Source: CAD feature listing. Evaluate the final solid. Frame: model axes, mm. A direction names the side the tool comes from. Round coordinates to 2 decimals unless told otherwise and drop trailing zeros. Loops run counter-clockwise (first coordinate to the right, second up) from the corner with the lowest first, then second, coordinate; pieces in that order, holes last. Notation, with made-up numbers: M -23.5,16.5 L -8.5,16.5 A27 ccw -8.5,55.5 Z; hole C 62.25,-11.75 d7. An arc over 180 degrees is marked long. One line per item, written item: value.
from build123d import *

# Parameters (mm, degrees)
ESBO_O1_W             = 8
ESBO_O1_H             = 8
CORTE_EXTRUS_O1_DEPTH = 46


with BuildPart() as part:
    # Sketch1 → Revolve1 (revolve)
    with BuildSketch(Plane.XY):
        with BuildLine():
            Line((0, -20), (0, -122))
            ThreePointArc((0, -122), (0.146446609, -122.353553391), (0.5, -122.5))
            Line((0.5, -122.5), (9.616336506, -122.5))
            ThreePointArc((9.616336506, -122.5), (9.920717221, -122.39667667), (10.099299419, -122.129409523))
            Line((10.099299419, -122.129409523), (12.679491924, -112.5))
            Line((12.679491924, -112.5), (22.320508076, -112.5))
            Line((22.320508076, -112.5), (24.900700581, -122.129409523))
            ThreePointArc((24.900700581, -122.129409523), (25.079282779, -122.39667667), (25.383663494, -122.5))
            Line((25.383663494, -122.5), (34.5, -122.5))
            ThreePointArc((34.5, -122.5), (34.853553391, -122.353553391), (35, -122))
            Line((35, -122), (35, -50))
            Line((35, -50), (44.5, -50))
            ThreePointArc((44.5, -50), (44.853553391, -49.853553391), (45, -49.5))
            Line((45, -49.5), (45, -10))
            Line((45, -10), (2.5, -10))
            Line((2.5, -10), (0, -20))
        make_face()
    revolve(axis=Axis((0, 0, 0), (1, 0, 0)))

    # Esboço1 → Corte-extrusão1 (cut, through all)
    with BuildSketch(Plane.ZY):
        with Locations((0, -10)):
            Rectangle(ESBO_O1_W, ESBO_O1_H)
    extrude(amount=-CORTE_EXTRUS_O1_DEPTH, mode=Mode.SUBTRACT)


solid = part.part
1. Reachability of faces 4 (the face through (2.344, 8.432, 6.465)), 5 (the face through (12.554, 24.489, 110.281)), 6 (the face through (23, -14, 0)) from +Z, -Z, +X, -X, +Y, -Y: full face, straight path, thin tool, end or side. Return the list, or none.
Report:
face 4: -X
face 5: none
face 6: +X, -X
2. Ray query, line 1 (Y direction, x = 20, z = 0); line 2 (Z direction, x = 36, y = 0); line 3 (Z direction, x = 14.5, y = 0). Return the intervals inside material, ascending. Write a range as [from, to].
Report:
line 1: y = [-112.5, -14], [10, 112.5]
line 2: z = [-50, -10], [10, 50]
line 3: z = [-112.5, -10], [10, 112.5]
3. Pull-direction query (Z, two-part tool) for faces 1 (the face through (35, 2, 53)), 2 (the face through (23, 10, 0)), 3 (the face through (39.82, -47.69, -15.02)); classes: released by +Z, released by -Z, zero draft, split by the parting line, or undercut.
Report:
face 1: zero draft
face 2: undercut
face 3: split by the parting line
4. Section query C-C (x = 6). Return the cut outline in (y, z).
Report:
outline: C 0,0 d245; hole M -14,-4 L -9.17,-4 A10 ccw long -9.17,4 L -14,4 Z
5. Section query D-D (x = 18.5). Return the cut outline in (y, z).
Report:
outline: C 0,0 d225; hole M -14,-4 L -9.17,-4 A10 ccw long -9.17,4 L -14,4 Z
6. Pin query (flat end, axial travel): pin 1 (10 mm diameter, centred on x = 25.5, z = -64, fed in from -Y); pin 2 (6 mm diameter, centred on x = 40, y = -91.5, fed in from -Z); pin 3 (8 mm diameter, centred on x = 30, y = -25.5, fed in from +Z); pin 4 (6 mm diameter, centred on x = 24, y = 66, fed in from -Z). Return the tip coordinate at first contact, or that it passes through.
Report:
pin 1: stops at y = -107.36
pin 2: passes through
pin 3: stops at z = 120.6
pin 4: stops at z = -104.87
